```python
from build123d import *

# Parameters (mm, degrees)
SKETCH1_R           = 0.75
BOSS_EXTRUDE1_DEPTH = 10
FILLET3_R           = 1
BOSS_EXTRUDE3_START = 2
SKETCH4_R           = 0.75
BOSS_EXTRUDE3_DEPTH = 2
SKETCH5_R           = 0.75
BOSS_EXTRUDE4_DEPTH = 2


with BuildPart() as part:
    # Sketch1 → Boss-Extrude1 (new body)
    with BuildSketch(Plane.XY):
        Circle(SKETCH1_R)
    extrude(amount=BOSS_EXTRUDE1_DEPTH)

    # Sketch3 → Revolve1 (revolve)
    with BuildSketch(Plane(origin=(0, 0, 0), x_dir=(0, 0, -1), z_dir=(1, 0, 0)), mode=Mode.PRIVATE) as revolve1_sk:
        Polygon((-3.5, 0), (-3.5, 2.5), (-5, 0), align=None)
    revolve1 = revolve(revolve1_sk.sketch.rotate(Axis((0, 0, 5), (0, 0, -1)), 270), axis=Axis((0, 0, 5), (0, 0, -1)))

    # Mirror1: Revolve1 across plane
    add(revolve1.mirror(Plane(origin=(0, 0, 5), x_dir=(1, 0, 0), z_dir=(0, 0, -1))))

    # Fillet3
    fillet3_edges = [part.edges().sort_by_distance(p)[0] for p in [
        (0, -0.75, 5.45),
    ]]
    fillet(fillet3_edges, radius=FILLET3_R)

    # Fillet4: read off the stored shape, not the designer's step
    # Fillet4 outline → Fillet4 (revolve)
    with BuildSketch(Plane.XZ):
        with BuildLine():
            Line((0.75, 4.883809621), (0.75, 4.278013821))
            Line((0.75, 4.278013821), (1.203310298, 4.278013821))
            ThreePointArc((1.203310298, 4.278013821), (0.917148948, 4.536383889), (0.75, 4.883809621))
        make_face()
    revolve(axis=Axis((0, 0, 0), (0, 0, 1)))

    # Sketch4 → Boss-Extrude3 (add)
    with BuildSketch(Plane(origin=(0, 0, 0), x_dir=(-1, 0, 0), z_dir=(0, 0, -1)).offset(BOSS_EXTRUDE3_START)):
        Circle(SKETCH4_R)
    extrude(amount=-BOSS_EXTRUDE3_DEPTH)

    # Sketch5 → Boss-Extrude4 (add)
    with BuildSketch(Plane.XY.offset(10)):
        with Locations(Location((0, 0, 0), (0, 0, 180))):
            Circle(SKETCH5_R)
    extrude(amount=BOSS_EXTRUDE4_DEPTH)


solid = part.part
```
Model file for the job. Use its own axes, mm. A direction names the side the tool comes from. Coordinates: 2 decimals unless noted, no trailing zeros. Write each loop counter-clockwise with the first axis right and the second up, starting at its lowest first coordinate (ties: lowest second). Pieces come first, ordered by that corner, then holes. Notation, with made-up numbers: (82.5, 87.5) - (137.5, 87.5) arc R24 ccw to (137.5, 102.5) - close; hole circle Ø7 at (32, 56). An arc over 180 degrees is marked (long way). Use a Markdown table: item, result. Add a question column.
Item 1: 3-axis set-ups, long thin cutter, end or side, ignore diameter. For faces 1 (the face through (0, 0, 12)), 2 (the face through (1, 1, 3.5)), 3 (the face through (1, 1, 6.5)): which of +Z, -Z, +X, -X, +Y, -Y reach the whole face in a straight line?
Item 2: Drop flat-ended pins along their axis: pin 1 (2 mm diameter, centred on x = -1, y = -1, fed in from -Z); pin 2 (1 mm diameter, centred on x = -0.5, y = 1.5, fed in from +Z). Give the stop position or say it passes through.
Item 3: Band-saw the part on A-A, the plane z = 8.75. Write the cut outline in (x, y), and give its area (3 significant figures).
Item 4: Drill centre lines: line 1 along Z through (x, y) = (-0.6, -1.15); line 2 along Z through (x, y) = (-0.9, -1.9); line 3 along X through (y, z) = (-0.05, 10.75). Where is each one in solid material? Low to high.
A:
| question | item | result |
|---|---|---|
| 1 | face 1 | +Z, +X, -X, +Y, -Y |
| 1 | face 2 | -Z |
| 1 | face 3 | +Z |
| 2 | pin 1 | stops at z = -2 |
| 2 | pin 2 | stops at z = 6.5 |
| 3 | outline | circle Ø1.5 at (0, 0) |
| 3 | area | 1.77 mm² |
| 4 | line 1 | z = 3.5 to 4.22, 5.78 to 6.5 |
| 4 | line 2 | z = 3.5 to 3.74, 6.26 to 6.5 |
| 4 | line 3 | x = -0.75 to 0.75 |
